from build123d import *

# Parameters (mm, degrees)
SCHIZZO4_R           = 38.5
CORPOCONTATTO_DEPTH  = 3
CORPOROTANTE_DEPTH   = 60.805
RACCORDO_R           = 10
SCHIZZO6_W           = 104.61
SCHIZZO6_H           = 90
TAGLIOCENTRALE_DEPTH = 31
SCHIZZO7_R           = 27.5
CONTATTO_DEPTH       = 2


with BuildPart() as part:
    # Schizzo4 → CorpoContatto (new body)
    with BuildSketch(Plane.XY):
        Circle(SCHIZZO4_R)
    extrude(amount=CORPOCONTATTO_DEPTH)

    # Schizzo5 → CorpoRotante (add, symmetric)
    with BuildSketch(Plane(origin=(0, 0, 0), x_dir=(1, 0, 0), z_dir=(0, 1, 0))):
        with BuildLine():
            Line((52.305, -3), (-52.305, -3))
            Line((-52.305, -3), (-52.305, -181))
            ThreePointArc((-52.305, -181), (-37.074552622, -217.769552622), (-0.305, -233))
            Line((-0.305, -233), (0.305, -233))
            ThreePointArc((0.305, -233), (37.074552622, -217.769552622), (52.305, -181))
            Line((52.305, -181), (52.305, -3))
        make_face()
    extrude(amount=CORPOROTANTE_DEPTH, both=True)

    # Raccordo
    raccordo_edges = [part.edges().sort_by_distance(p)[0] for p in [
        (52.305, -60.805, 92),
        (-52.305, -60.805, 92),
        (-37.074552622, -60.805, 217.769552622),
        (0, -60.805, 233),
        (37.074552622, -60.805, 217.769552622),
        (52.305, 60.805, 92),
        (-52.305, 60.805, 92),
        (-37.074552622, 60.805, 217.769552622),
        (0, 60.805, 233),
        (37.074552622, 60.805, 217.769552622),
    ]]
    fillet(raccordo_edges, radius=RACCORDO_R)

    # Schizzo6 → TaglioCentrale (cut, symmetric)
    with BuildSketch(Plane(origin=(0, 0, 0), x_dir=(1, 0, 0), z_dir=(0, 1, 0))):
        with Locations((0, -188)):
            Rectangle(SCHIZZO6_W, SCHIZZO6_H)
    extrude(amount=TAGLIOCENTRALE_DEPTH, both=True, mode=Mode.SUBTRACT)

    # Schizzo7 → Contatto (add)
    with BuildSketch(Plane.XZ.offset(-31)):
        with Locations(Location((0, 187, 0), (0, 0, 90))):
            Circle(SCHIZZO7_R)
    contatto = extrude(amount=CONTATTO_DEPTH)

    # Specchia1: Contatto across plane
    add(contatto.mirror(Plane.ZX))


solid = part.part
Source: CAD feature listing. Evaluate the final solid. Frame: model axes, mm. A direction names the side the tool comes from. Coordinates: 2 decimals unless noted, no trailing zeros. Loops run counter-clockwise (first coordinate to the right, second up) from the corner with the lowest first, then second, coordinate; pieces in that order, holes last. Notation, with made-up numbers: (-1.75, -15.75) - (5.25, -15.75) arc R13 cw to (5.25, -3.75) - close; hole circle Ø3 at (70, -3.5). An arc over 180 degrees is marked (long way). One line per question, with ' | ' between items.
1) Set-up query: faces 4 (the face through (1, 41, 3)), 5 (the face through (-1, 31, 157)), 6 (the face through (0, 29, 187)). Return all of +Z, -Z, +X, -X, +Y, -Y with unobstructed straight access to the full face (end or side cutting, diameter ignored); none if empty.
Report:
face 4: -Z | face 5: none | face 6: +Z, +X, -X
2) Pull-direction query (Y, two-part tool) for faces 1 (the face through (49.3, -57.95, 90.75)), 2 (the face through (-30.55, -23.43, 1.48)), 3 (the face through (10.533, -30.014, 212.403)); classes: released by +Y, released by -Y, zero draft, split by the parting line, or undercut.
Report:
face 1: released by -Y | face 2: split by the parting line | face 3: undercut
3) Section A-A, the plane y = 0. Return loops of the section in (x, z) (3 decimals).
Report:
outline: (-52.305, 3) - (-38.5, 3) - (-38.5, 0) - (38.5, 0) - (38.5, 3) - (52.305, 3) - (52.305, 143) - (-52.305, 143) - close
4) Section C-C, the plane y = -15. Return loops of the section in (x, z) (3 decimals).
Report:
outline: (-52.305, 3) - (-35.458, 3) - (-35.458, 0) - (35.458, 0) - (35.458, 3) - (52.305, 3) - (52.305, 143) - (-52.305, 143) - close
5) Section B-B, the plane y = 36. Return loops of the section in (x, z) (3 decimals).
Report:
outline: (-52.305, 3) - (-13.647, 3) - (-13.647, 0) - (13.647, 0) - (13.647, 3) - (52.305, 3) - (52.305, 181) arc R52 ccw to (0.305, 233) - (-0.305, 233) arc R52 ccw to (-52.305, 181) - close
6) First-contact query: P1, Ø3, axis at x = -14.5, y = 44, coming from the -Z side; P2, Ø8, axis at x = 13.5, y = 39.5, coming from the +Z side; P3, Ø4, axis at x = 17.5, y = 33, coming from the +Z side. Flat tips, straight axial feed; report the tip coordinate or a pass-through.
Report:
P1: stops at z = 3 | P2: stops at z = 232.18 | P3: stops at z = 230.73
7) Line query: line 1 along Y through (x, z) = (-4.5, 168.5) (3 decimals); line 2 along Y through (x, z) = (-19.5, 218.5); line 3 along Z through (x, y) = (-43, 14). Output: solid intervals per line, ascending.
Report:
line 1: y = -60.805 to -29, 29 to 60.805 | line 2: y = -60.8 to -31, 31 to 60.8 | line 3: z = 3 to 143
